Check sheet for the modelled part. Datum: model origin and axes. Units: mm. Face numbers are marked on the shaded views. A direction names the side the tool comes from. Round coordinates to 2 decimals unless told otherwise and drop trailing zeros. Order: outer loops, then holes, each group sorted by start corner. A loop starts at its lowest first (then second) coordinate and runs counter-clockwise, first axis right, second up. Notation, with made-up numbers: (7, 86) -> (39, 86) arc R24 cw to (39, 100) -> close; hole circle Ø5 at (-1.5, 6.5). An arc over 180 degrees is marked (long way). Answer in a Markdown table with one row per item. Add a question column.
1. Draft check along X on the marked faces 1, 2 and 3. Enter one of: +X half, -X half, draft (parallel to the pull), parting line (faces both ways), or undercut.
2. Sectioned sample at B-B, the plane y = -4. Record the boundary of the cut face in (x, z), then the cut area to 3 significant figures.
3. Sectioned sample at A-A, the plane x = -11. Record the boundary of the cut face in (y, z).
4. Sectioned sample at D-D, the plane z = 9. Record the boundary of the cut face in (x, y), then the cut area to 3 significant figures.
5. Access from +Z, -Z, +X, -X, +Y, -Y to the whole of each face (thin tool, end or side, straight path). Record for the marked faces 4 and 5.
6. Sectioned sample at C-C, the plane y = 8.5. Record the boundary of the cut face in (x, z).
7. Material ranges on L1, parallel to X at y = -9, z = 4; L2, parallel to Y at x = 9.5, z = 6; L3, parallel to X at y = -4.5, z = 0.5, recorded low to high. Write a range as from..to.
8. Depth check by flat-ended pin: P1, Ø2, axis at x = 1.5, z = 3, coming from the -Y side; P2, Ø3, axis at y = -11.5, z = 1, coming from the +X side; P3, Ø3, axis at x = -17.5, z = 1.5, coming from the +Y side. Enter the tip coordinate at first touch or a pass-through.
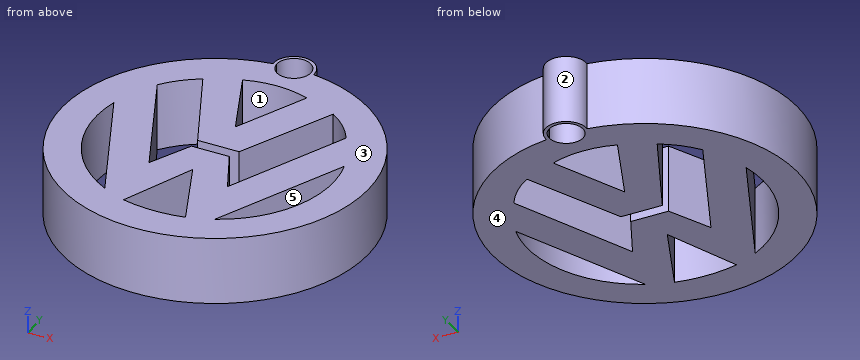
```python
from build123d import *

# Parameters (mm, degrees)
F1_DEPTH = 10


with BuildPart() as f1:
    # F0 (on Top) → F1 (new body)
    with BuildSketch(Plane.XY):
        with BuildLine():
            ThreePointArc((2.497035, 22.477096), (0.016859, 20.098873), (-2.495166, 22.44343))
            ThreePointArc((-2.495166, 22.44343), (-2.743734, 22.412651), (-2.991944, 22.379114))
            ThreePointArc((-2.991944, 22.379114), (0.304191, -22.508373), (2.994635, 22.419486))
            ThreePointArc((2.994635, 22.419486), (2.745995, 22.449673), (2.497035, 22.477096))
        make_face()
        with BuildLine():
            ThreePointArc((4.713637, -17.017649), (0.09357, -17.47788), (-4.514231, -16.907794))
            Line((-4.514231, -16.907794), (0, -5.973655))
            Line((0, -5.973655), (4.713637, -17.017649))
        make_face(mode=Mode.SUBTRACT)
        with BuildLine():
            ThreePointArc((-8.029609, -15.479672), (-15.820727, -7.22331), (-16.927909, 4.074618))
            Line((-16.927909, 4.074618), (-8.029609, -15.479672))
        make_face(mode=Mode.SUBTRACT)
        with BuildLine():
            ThreePointArc((17.23717, 3.964762), (16.349809, -7.479071), (8.33887, -15.699385))
            Line((8.33887, -15.699385), (17.23717, 3.964762))
        make_face(mode=Mode.SUBTRACT)
        with BuildLine():
            ThreePointArc((-13.96181, 10.665952), (-11.867447, 12.939615), (-9.347876, 14.730607))
            Line((-9.347876, 14.730607), (-2.811192, 0.784471))
            Line((-2.811192, 0.784471), (3.325497, 0.784471))
            Line((3.325497, 0.784471), (9.876846, 14.840462))
            ThreePointArc((9.876846, 14.840462), (12.296267, 12.852136), (14.161215, 10.336385))
            Line((14.161215, 10.336385), (6.031903, -7.679928))
            Line((6.031903, -7.679928), (2.736236, -0.868883))
            Line((2.736236, -0.868883), (-2.866398, -0.868883))
            Line((-2.866398, -0.868883), (-5.876908, -7.100868))
            Line((-5.876908, -7.100868), (-13.96181, 10.665952))
        make_face(mode=Mode.SUBTRACT)
        with BuildLine():
            ThreePointArc((-4.624086, 16.927719), (0.16409, 17.695766), (4.933347, 16.817864))
            Line((4.933347, 16.817864), (0, 6.066685))
            Line((0, 6.066685), (-4.624086, 16.927719))
        make_face(mode=Mode.SUBTRACT)
        with BuildLine():
            ThreePointArc((-2.991944, 22.379114), (-2.743734, 22.412651), (-2.495166, 22.44343))
            ThreePointArc((-2.495166, 22.44343), (-0.07773, 25.097607), (2.5, 22.598816))
            ThreePointArc((2.5, 22.598816), (2.499259, 22.537938), (2.497035, 22.477096))
            ThreePointArc((2.497035, 22.477096), (2.745995, 22.449673), (2.994635, 22.419486))
            ThreePointArc((2.994635, 22.419486), (-0.020231, 25.598748), (-2.991944, 22.379114))
        make_face()
    extrude(amount=F1_DEPTH)


solid = f1.part
```
Answer key:
| question | item | result |
|---|---|---|
| 1 | face 1 | undercut |
| 1 | face 2 | parting line |
| 1 | face 3 | draft |
| 2 | outline | (-22.04, 0) -> (-16.92, 0) -> (-16.92, 10) -> (-22.04, 10) -> close; (-13.25, 0) -> (-7.29, 0) -> (-7.29, 10) -> (-13.25, 10) -> close; (-4.38, 0) -> (4.25, 0) -> (4.25, 10) -> (-4.38, 10) -> close; (7.69, 0) -> (13.63, 0) -> (13.63, 10) -> (7.69, 10) -> close; (17.49, 0) -> (22.34, 0) -> (22.34, 10) -> (17.49, 10) -> close |
| 2 | area | 305 mm² |
| 3 | outline | (-19.56, 0) -> (-13.5, 0) -> (-13.5, 10) -> (-19.56, 10) -> close; (-8.95, 0) -> (4.16, 0) -> (4.16, 10) -> (-8.95, 10) -> close; (13.65, 0) -> (19.65, 0) -> (19.65, 10) -> (13.65, 10) -> close |
| 4 | outline | (-2.99, 22.38) arc R22.55 ccw (long way) to (2.99, 22.42) arc R3 ccw (long way) to start; hole (-16.93, 4.07) arc R17.55 ccw to (-8.03, -15.48) -> close; hole (-13.96, 10.67) -> (-5.88, -7.1) -> (-2.87, -0.87) -> (2.74, -0.87) -> (6.03, -7.68) -> (14.16, 10.34) arc R12.82 ccw to (9.88, 14.84) -> (3.33, 0.78) -> (-2.81, 0.78) -> (-9.35, 14.73) arc R14.86 ccw to start; hole (-4.62, 16.93) -> (0, 6.07) -> (4.93, 16.82) arc R14.29 ccw to start; hole (-4.51, -16.91) arc R20.92 ccw to (4.71, -17.02) -> (0, -5.97) -> close; hole (2.5, 22.48) arc R2.5 ccw to (2.5, 22.6) arc R2.5 ccw (long way) to start; hole (8.34, -15.7) arc R16.85 ccw to (17.24, 3.96) -> close |
| 4 | area | 1,140 mm² |
| 5 | face 4 | -Z, +X, -X, +Y, -Y |
| 5 | face 5 | +Z, -Z |
| 6 | outline | (-20.76, 0) -> (-12.98, 0) -> (-12.98, 10) -> (-20.76, 10) -> close; (-6.43, 0) -> (-1.04, 0) -> (-1.04, 10) -> (-6.43, 10) -> close; (1.12, 0) -> (6.92, 0) -> (6.92, 10) -> (1.12, 10) -> close; (13.33, 0) -> (21.06, 0) -> (21.06, 10) -> (13.33, 10) -> close |
| 7 | L1 | x = -20.51..-14.89, -10.98..-1.25, 1.29..11.37, 15.57..20.81 |
| 7 | L2 | y = -20.48..-15.08, -13.13..0.01, 14.03..20.57 |
| 7 | L3 | x = -21.94..-16.8, -13.03..-7.06, -4.62..4.49, 7.47..13.41, 17.37..22.24 |
| 8 | P1 | stops at y = -22.51 |
| 8 | P2 | stops at x = 20.35 |
| 8 | P3 | stops at y = 15.79 |
